Could you check a few things on this model? Use its own coordinates, in mm. Give positions to 0.01 mm unless a question says otherwise; leave off trailing zeros. Write each loop counter-clockwise with the first axis right and the second up, starting at its lowest first coordinate (ties: lowest second). Pieces come first, ordered by that corner, then holes. Notation, with made-up numbers: (46, 57) - (99, 57) arc R20 cw to (99, 65) - close; hole circle Ø5 at (88, 73.5). An arc over 180 degrees is marked (long way). Write item = value, one per line.
from build123d import *

# Parameters (mm, degrees)
BOSS_EXTRU_1_DEPTH              = 1
EXTRU_MINCE1_DEPTH              = 1.5
EXTRU_MINCE1_TAPER              = -10
ENL_V_DE_MAT_EXTRU_MINCE1_DEPTH = 3.5000001
ESQUISSE4_R                     = 2.5
BOSS_EXTRU_2_DEPTH              = 3.8


with BuildPart() as part:
    # Esquisse1 → Boss.-Extru.1 (new body)
    with BuildSketch(Plane.XY):
        Polygon((-84.524791386, -59.467077727), (2.7, -59.467077727), (84.524791386, -59.467077727), (93.762395693, -43.467077727), (68.666666667, 0), (-68.666666667, 0), (-93.762395693, -43.467077727), align=None)
    extrude(amount=BOSS_EXTRU_1_DEPTH)

    # Esquisse2 → Extru.-Mince1 (add)
    with BuildSketch(Plane.XY.offset(1)):
        Polygon((-93.762395693, -43.467077727), (-84.524791386, -59.467077727), (84.524791386, -59.467077727), (93.762395693, -43.467077727), (68.666666667, 0), (-68.666666667, 0), align=None)
        Polygon((-91.683934724, -43.467077727), (-83.485560901, -57.667077727), (83.485560901, -57.667077727), (91.683934724, -43.467077727), (67.627436182, -1.8), (-67.627436182, -1.8), align=None, mode=Mode.SUBTRACT)
    extrude(amount=EXTRU_MINCE1_DEPTH, taper=EXTRU_MINCE1_TAPER)

    # Esquisse3 → Enlèv. de mat.-Extru.-Mince1 (cut, through all)
    with BuildSketch(Plane(origin=(0, 0, 0), x_dir=(-1, 0, 0), z_dir=(0, 0, -1))):
        Polygon((85.621756897, -61.367077727), (95.956326716, -43.467077727), (69.763632178, 1.9), (-69.763632178, 1.9), (-95.956326716, -43.467077727), (-85.621756897, -61.367077727), align=None)
        Polygon((84.524791386, -59.467077727), (93.762395693, -43.467077727), (68.666666667, 0), (-68.666666667, 0), (-93.762395693, -43.467077727), (-84.524791386, -59.467077727), align=None, mode=Mode.SUBTRACT)
    extrude(amount=-ENL_V_DE_MAT_EXTRU_MINCE1_DEPTH, mode=Mode.SUBTRACT)

    # Esquisse4 → Boss.-Extru.2 (add)
    with BuildSketch(Plane.XY.offset(1)):
        with Locations((25.665479371, -13.424541306)):
            Circle(ESQUISSE4_R)
    extrude(amount=BOSS_EXTRU_2_DEPTH)


solid = part.part
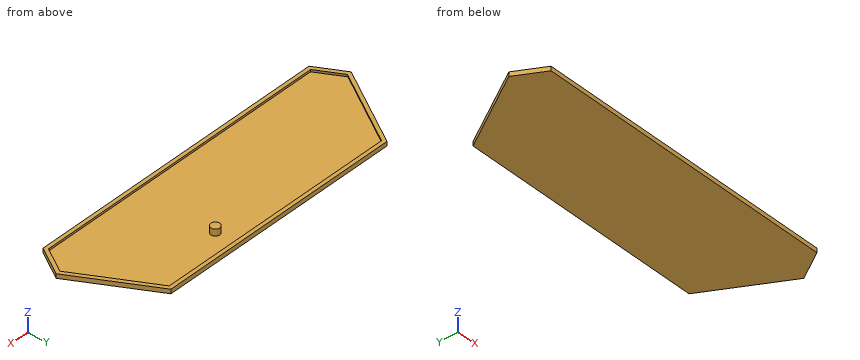
1. If we section it at A-A, the plane z = 3.6: Please give me the cut outline in (x, y), and give its area (3 significant figures).
Filled sheet:
outline = circle Ø5 at (25.67, -13.42)
area = 19.6 mm2
2. For pin 1 (8 mm diameter, centred on x = 50.5, y = -13, fed in from +Z); pin 2 (1.5 mm diameter, centred on y = -10.5, z = 1, fed in from +X); pin 3 (2 mm diameter, centred on y = -6.5, z = 2.5, fed in from +X); pin 4 (10 mm diameter, centred on x = 1.5, y = -30.5, fed in from -Z), each with a flat end and sliding along its axis, tell me the tip position at first contact or that it passes through.
Filled sheet:
pin_1 = 1
pin_2 = 75.16
pin_3 = 73
pin_4 = 0
3. I need wall thicknesses on line 1 (Y direction, x = -44, z = 2.4); line 2 (Y direction, x = -7, z = 2.45); line 3 (Z direction, x = 6, y = -17.5). Which ranges of each line are inside material? Lowest first, please.
Filled sheet:
line_1 = -59.47 to -57.42, -2.05 to 0
line_2 = -59.47 to -57.41, -2.06 to 0
line_3 = 0 to 1
